The drawing under review shows one solid part. Ordinate dimensions are in mm from its lowest x, y, z. A direction names the side the tool comes from. Coordinates: 2 decimals unless noted, no trailing zeros. Order: outer loops, then holes, each group sorted by start corner. A loop starts at its lowest first (then second) coordinate and runs counter-clockwise, first axis right, second up. Notation, with made-up numbers: (44.5, 62) - (96.5, 62) arc R19 cw to (96.5, 78) - close; hole circle Ø2 at (74, 85). An arc over 180 degrees is marked (long way). Answer in a Markdown table with one row per item.
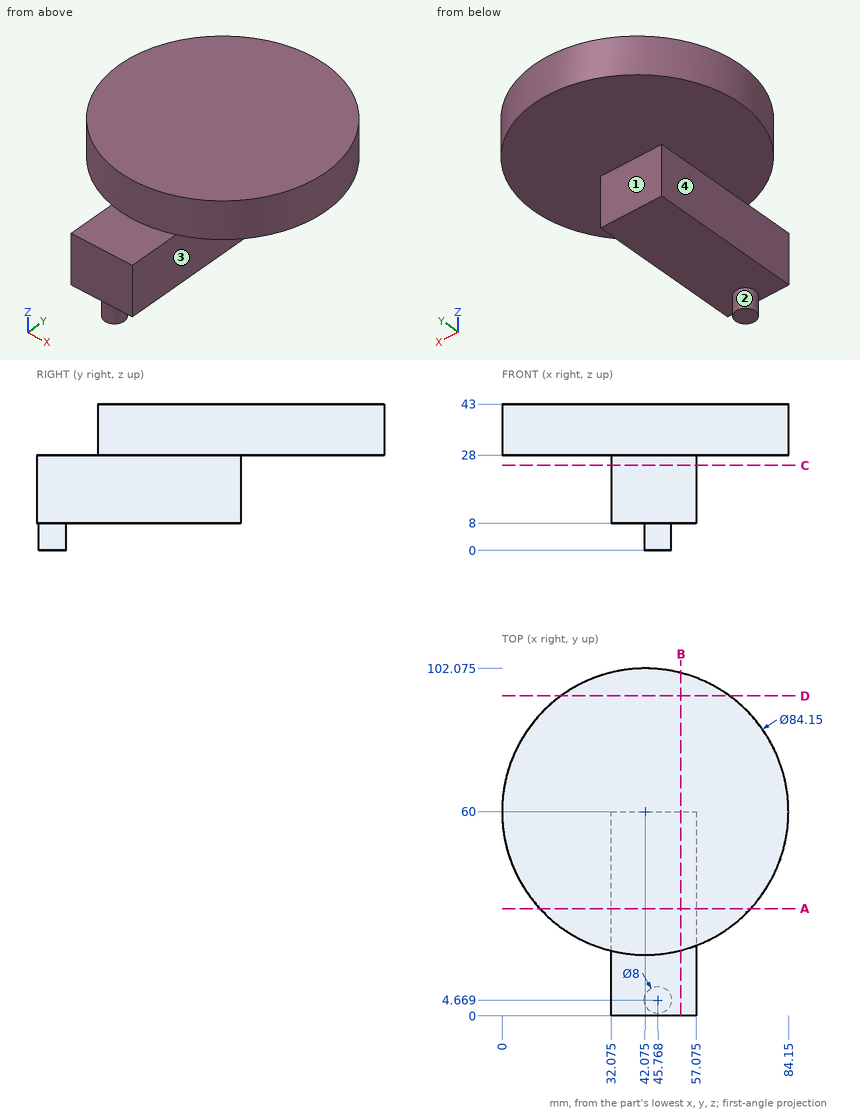
Item 1: We need section B-B, the plane x = 52.5. Write out the cut boundary in (y, z).
Check values:
| item | result |
|---|---|
| outline | (0, 8) - (60, 8) - (60, 28) - (100.76, 28) - (100.76, 43) - (19.24, 43) - (19.24, 28) - (0, 28) - close |
Item 2: To check wall thickness, follow line 1 (Y direction, x = 42, z = 41) (1 decimal); line 2 (Z direction, x = 26, y = 84); line 3 (X direction, y = 41, z = 12) (3 decimals). State the ranges of each line that lie inside material, in increasing order. Write a range as from..to.
Check values:
| item | result |
|---|---|
| line 1 | 17.9..102.1 |
| line 2 | 28..43 |
| line 3 | 32.075..57.075 |
Item 3: Clearance check with flat-ended pins moving along their axes: pin 1 Ø1 at (y, z) = (76.5, 31.5) entering from -X; pin 2 Ø1.5 at (x, y) = (31.5, 15) entering from +Z; pin 3 Ø12 at (x, z) = (46, 13.5) entering from +Y. State where each tip first meets the part, or that it passes through.
Check values:
| item | result |
|---|---|
| pin 1 | x = 3.16 |
| pin 2 | z = 28 |
| pin 3 | y = 60 |
Item 4: We need section C-C, the plane z = 25. Write out the cut boundary in (x, y) (3 decimals), then the cut area to 3 significant figures.
Check values:
| item | result |
|---|---|
| outline | (32.075, 0) - (57.075, 0) - (57.075, 60) - (32.075, 60) - close |
| area | 1,500 mm^2 |
Item 5: Tool access review of the marked faces 1, 2, 3 and 4: name each direction out of +Z, -Z, +X, -X, +Y, -Y from which nothing blocks a thin tool from reaching the whole face with its end or side.
Check values:
| item | result |
|---|---|
| face 1 | -Z, +X, -X, +Y |
| face 2 | -Z |
| face 3 | -Z, +X, +Y, -Y |
| face 4 | -Z, -X, +Y, -Y |
Item 6: We need section A-A, the plane y = 31.5. Write out the cut boundary in (x, z) (1 decimal), then the cut area to 3 significant figures.
Check values:
| item | result |
|---|---|
| outline | (11.1, 28) - (32.1, 28) - (32.1, 8) - (57.1, 8) - (57.1, 28) - (73, 28) - (73, 43) - (11.1, 43) - close |
| area | 1,430 mm^2 |
Item 7: We need section D-D, the plane y = 94. Write out the cut boundary in (x, z).
Check values:
| item | result |
|---|---|
| outline | (17.29, 28) - (66.86, 28) - (66.86, 43) - (17.29, 43) - close |
